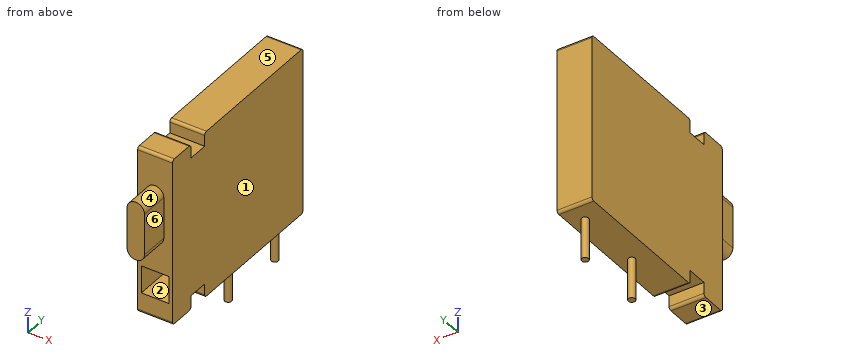
```python
from build123d import *

# Parameters (mm, degrees)
SKETCH_1_W          = 2.54
SKETCH_1_H          = 14.2
EXTRUDE_1_DEPTH     = 12.2
SKETCH_2_R          = 0.25
EXTRUDE_2_DEPTH     = 3
EXTRUDE_3_DEPTH     = 2.1
SKETCH_4_W          = 2
SKETCH_4_H          = 2
CUT_EXTRUDE_1_DEPTH = 5
CUT_EXTRUDE_2_REACH = 20.893
SKETCH_5_W          = 2.597491907
SKETCH_5_H          = 1.5
SKETCH_5_W_2        = 2.655260115
FILLET_1_R          = 0.2


with BuildPart() as part:
    # 草图1 → 凸台-拉伸1 (new body)
    with BuildSketch(Plane.XY):
        with Locations((1.27, 7.1)):
            Rectangle(SKETCH_1_W, SKETCH_1_H)
    extrude(amount=EXTRUDE_1_DEPTH)

    # 草图2 → 凸台-拉伸2 (add)
    with BuildSketch(Plane(origin=(0, 0, 0), x_dir=(-1, 0, 0), z_dir=(0, 0, -1))):
        with Locations((-1.5, 12.7)):
            Circle(SKETCH_2_R)
        with Locations((-1.5, 7.62)):
            Circle(SKETCH_2_R)
    extrude(amount=EXTRUDE_2_DEPTH)

    # 草图3 → 凸台-拉伸3 (add)
    with BuildSketch(Plane(origin=(0, 0, 0), x_dir=(-1, 0, 0), z_dir=(0, -1, 0))):
        with BuildLine():
            Line((-1.905, -9.2), (-1.905, -6.2))
            ThreePointArc((-1.905, -6.2), (-1.27, -5.565), (-0.635, -6.2))
            Line((-0.635, -6.2), (-0.635, -9.2))
            ThreePointArc((-0.635, -9.2), (-1.27, -9.835), (-1.905, -9.2))
        make_face()
    extrude(amount=EXTRUDE_3_DEPTH)

    # 草图4 → 切除-拉伸1 (cut)
    with BuildSketch(Plane.XZ):
        with Locations((1.27, 2.5)):
            Rectangle(SKETCH_4_W, SKETCH_4_H)
    extrude(amount=-CUT_EXTRUDE_1_DEPTH, mode=Mode.SUBTRACT)

    # 草图5 → 切除-拉伸2 (cut, up to next)
    with BuildSketch(Plane(origin=(2.54, 0, 0), x_dir=(0, 0, -1), z_dir=(1, 0, 0)), mode=Mode.PRIVATE) as cut_extrude_2_sk1:
        with Locations((-12.498745954, 2.75)):
            Rectangle(SKETCH_5_W, SKETCH_5_H)
    cut_extrude_2_tool1 = extrude(cut_extrude_2_sk1.sketch, amount=-CUT_EXTRUDE_2_REACH, mode=Mode.PRIVATE) & part.part
    # 草图5 → 切除-拉伸2 (cut, up to next)
    with BuildSketch(Plane(origin=(2.54, 0, 0), x_dir=(0, 0, -1), z_dir=(1, 0, 0)), mode=Mode.PRIVATE) as cut_extrude_2_sk2:
        with Locations((0.327630058, 2.75)):
            Rectangle(SKETCH_5_W_2, SKETCH_5_H)
    cut_extrude_2_tool2 = extrude(cut_extrude_2_sk2.sketch, amount=-CUT_EXTRUDE_2_REACH, mode=Mode.PRIVATE) & part.part
    add(cut_extrude_2_tool1.solids().sort_by_distance((2.54, 2.75, 12.498746))[0], mode=Mode.SUBTRACT)
    add(cut_extrude_2_tool2.solids().sort_by_distance((2.54, 2.75, -0.32763))[0], mode=Mode.SUBTRACT)

    # 圆角1
    fillet_1_edges = [part.edges().sort_by_distance(p)[0] for p in [
        (1.27, 14.2, 12.2),
        (1.27, 14.2, 0),
        (1.27, 0, 0),
        (1.27, 3.5, 12.2),
        (1.27, 2, 12.2),
        (1.27, 3.5, 0),
        (1.27, 2, 0),
        (1.27, 0, 12.2),
    ]]
    fillet(fillet_1_edges, radius=FILLET_1_R)


solid = part.part
```
Geometry check sheet. Reference: the model listing, model coordinates, mm. Face numbers are marked on the shaded views. A direction names the side the tool comes from. Coordinates: 2 decimals unless noted, no trailing zeros. Order: outer loops, then holes, each group sorted by start corner. A loop starts at its lowest first (then second) coordinate and runs counter-clockwise, first axis right, second up.
Q1. Draft check along X on the marked faces 1, 2, 3 and 4. Enter one of: released by +X, released by -X, zero draft, split by the parting line, or undercut.
Reply:
face 1: released by +X
face 2: undercut
face 3: zero draft
face 4: split by the parting line
Q2. Sectioned sample at B-B on z = 3.25. Record the cut outline in (x, y).
Reply:
outline: (0, 0) - (0.27, 0) - (0.27, 5) - (2.27, 5) - (2.27, 0) - (2.54, 0) - (2.54, 14.2) - (0, 14.2) - close
Q3. Sectioned sample at C-C on y = 12.7. Record the cut outline in (x, z).
Reply:
outline: (0, 0) - (1.25, 0) - (1.25, -3) - (1.75, -3) - (1.75, 0) - (2.54, 0) - (2.54, 12.2) - (0, 12.2) - close
Q4. Sectioned sample at D-D on x = 0.95. Record the cut outline in (y, z), and give its area (3 significant figures).
Reply:
outline: (-2.1, 5.65) - (0, 5.65) - (0, 3.5) - (5, 3.5) - (5, 1.5) - (0, 1.5) - (0, 0.2) arc R0.2 ccw to (0.2, 0) - (1.8, 0) arc R0.2 ccw to (2, 0.2) - (2, 1) - (3.5, 1) - (3.5, 0.2) arc R0.2 ccw to (3.7, 0) - (14, 0) arc R0.2 ccw to (14.2, 0.2) - (14.2, 12) arc R0.2 ccw to (14, 12.2) - (3.7, 12.2) arc R0.2 ccw to (3.5, 12) - (3.5, 11.2) - (2, 11.2) - (2, 12) arc R0.2 ccw to (1.8, 12.2) - (0.2, 12.2) arc R0.2 ccw to (0, 12) - (0, 9.75) - (-2.1, 9.75) - close
area: 169 mm2
Q5. Depth check by flat-ended pin: pin 1 Ø0.6 at (x, z) = (0.5, 11.5) entering from -Y; pin 2 Ø0.8 at (x, y) = (2, 3) entering from +Z; pin 3 Ø0.6 at (y, z) = (-1.5, 8.5) entering from -X (3 decimals). Enter the tip coordinate at first touch or a pass-through.
Reply:
pin 1: stops at y = 0
pin 2: stops at z = 11.2
pin 3: stops at x = 0.635
Q6. Thickness scan on probe 1 along Z at (x, y) = (2.1, 1.75); probe 2 along Y at (x, z) = (0.8, 4.75); probe 3 along Z at (x, y) = (2, 11). Record the ranges inside material, lowest first.
Reply:
probe 1: z = 0 to 1.5, 3.5 to 12.2
probe 2: y = 0 to 14.2
probe 3: z = 0 to 12.2
Q7. Tool access check on the marked faces 5 and 6. Record the directions out of +Z, -Z, +X, -X, +Y, -Y that give a thin tool (end or side, any length) a straight path to the whole face; none if there is none.
Reply:
face 5: +Z, +X, -X, +Y, -Y
face 6: +Z, -Z, +X, -Y
Q8. Sectioned sample at A-A on y = 2.25. Record the cut outline in (x, z), and give its area (3 significant figures).
Reply:
outline: (0, 1) - (2.54, 1) - (2.54, 11.2) - (0, 11.2) - close; hole (0.27, 1.5) - (2.27, 1.5) - (2.27, 3.5) - (0.27, 3.5) - close
area: 21.9 mm2
